```python
from build123d import *

# Parameters (mm, degrees)
F0_R     = 15.644547
F0_R_2   = 15.650853
F0_R_3   = 15.947198
F0_R_4   = 15.533086
F1_DEPTH = 25.4


with BuildPart() as f1:
    # F0 (on Front) → F1 (new body)
    with BuildSketch(Plane.XZ):
        with BuildLine():
            ThreePointArc((11.669454, 17.846526), (0, 56.631885), (-11.669454, 17.846526))
            ThreePointArc((-11.669454, 17.846526), (-18.913895, 9.845772), (-21.312332, -0.677605))
            ThreePointArc((-21.312332, -0.677605), (-47.332079, -34.622215), (-7.100958, -20.105995))
            ThreePointArc((-7.100958, -20.105995), (-0.551606, -21.315965), (6.05156, -20.446351))
            ThreePointArc((6.05156, -20.446351), (44.238676, -37.166309), (21.183635, -2.434797))
            ThreePointArc((21.183635, -2.434797), (19.304517, 9.055951), (11.669454, 17.846526))
        make_face()
        with Locations((-29.344995, -21.465119)):
            Circle(F0_R, mode=Mode.SUBTRACT)
        with Locations((27.60382, -23.190841)):
            Circle(F0_R_2, mode=Mode.SUBTRACT)
        Circle(F0_R_3, mode=Mode.SUBTRACT)
        with Locations((0, 35.483696)):
            Circle(F0_R_4, mode=Mode.SUBTRACT)
    extrude(amount=F1_DEPTH)


solid = f1.part
```
Model file for the job. Use its own axes, mm. Coordinates: 2 decimals unless noted, no trailing zeros. Write each loop counter-clockwise with the first axis right and the second up, starting at its lowest first coordinate (ties: lowest second). Pieces come first, ordered by that corner, then holes. Notation, with made-up numbers: (71, 42.25) - (116, 42.25) arc R20 ccw to (116, 49.25) - close; hole circle Ø1 at (-15.5, 53). An arc over 180 degrees is marked (long way). Use a Markdown table: item, result. Add a question column.
Item 1: Drop flat-ended pins along their axis: pin 1 (2 mm diameter, centred on y = -8, z = 36.5, fed in from +X); pin 2 (4 mm diameter, centred on x = 34, y = -15, fed in from +Z); pin 3 (5 mm diameter, centred on y = -21.5, z = 8, fed in from +X). Give the stop position or say it passes through.
Item 2: Drill centre lines: line 1 along Z through (x, y) = (0, -9.25); line 2 along Z through (x, y) = (-3, -1.25); line 3 along X through (y, z) = (-23.5, -32). Where is each one in solid material? Low to high.
Item 3: Band-saw the part on A-A, the plane x = 0. Write the cut outline in (y, z).
Item 4: Band-saw the part on C-C, the plane x = -22.5. Write the cut outline in (y, z), and give its area (3 significant figures).
Item 5: Band-saw the part on B-B, the plane z = 28. Write the cut outline in (x, y), and give its area (3 significant figures).
Item 6: Two-plate mould, pull along X, no slides. Class faces 1 (the face through (-47.79, -12.52, -33.97)), 2 (the face through (-0.645, -12.522, -21.313)), 3 (the face through (-1.4, -25.4, -16.5)): pulls with the +X half, pulls with the -X half, needs draft (parallel to the pull), parting line crosses it, or undercut.
Item 7: Band-saw the part on D-D, the plane y = -13.75. Write the cut outline in (x, z) (3 decimals), and give its area (3 significant figures).
A:
| question | item | result |
|---|---|---|
| 1 | pin 1 | stops at x = 21.15 |
| 1 | pin 2 | stops at z = -1.91 |
| 1 | pin 3 | stops at x = 20.6 |
| 2 | line 1 | z = -21.32 to -15.95, 15.95 to 19.95, 51.02 to 56.63 |
| 2 | line 2 | z = -21.11 to -15.66, 15.66 to 20.24, 50.72 to 56.42 |
| 2 | line 3 | x = -48.98 to -40.91, -17.78 to -9.71, 7.74 to 14.67, 40.54 to 47.46 |
| 3 | outline | (-25.4, -21.32) - (0, -21.32) - (0, -15.95) - (-25.4, -15.95) - close; (-25.4, 15.95) - (0, 15.95) - (0, 19.95) - (-25.4, 19.95) - close; (-25.4, 51.02) - (0, 51.02) - (0, 56.63) - (-25.4, 56.63) - close |
| 4 | outline | (-25.4, -42.67) - (0, -42.67) - (0, -35.53) - (-25.4, -35.53) - close; (-25.4, -7.4) - (0, -7.4) - (0, -0.26) - (-25.4, -0.26) - close |
| 4 | area | 363 mm² |
| 5 | outline | (-19.78, -25.4) - (-13.61, -25.4) - (-13.61, 0) - (-19.78, 0) - close; (13.61, -25.4) - (19.78, -25.4) - (19.78, 0) - (13.61, 0) - close |
| 5 | area | 313 mm² |
| 6 | face 1 | undercut |
| 6 | face 2 | undercut |
| 6 | face 3 | needs draft |
| 7 | outline | (-21.312, -0.678) arc R22.286 ccw (long way) to (-7.101, -20.106) arc R21.323 ccw to (6.052, -20.446) arc R21.726 ccw (long way) to (21.184, -2.435) arc R21.323 ccw to (11.669, 17.847) arc R21.148 ccw (long way) to (-11.669, 17.847) arc R21.323 ccw to start; hole circle Ø31.289 at (-29.345, -21.465); hole circle Ø31.894 at (0, 0); hole circle Ø31.066 at (0, 35.484); hole circle Ø31.302 at (27.604, -23.191) |
| 7 | area | 2,440 mm² |
